Autodesk Inventor part; units mm, degrees
ref_plane "YZ Plane" through (0, 0, 0) normal (1, 0, 0) x (0, 1, 0)
ref_plane "XZ Plane" through (0, 0, 0) normal (0, 1, 0) x (-1, 0, 0)
ref_plane "XY Plane" through (0, 0, 0) normal (0, 0, 1) x (1, 0, 0)
sketch "Sketch1" plane through (0, 0, 0) normal (0, 1, 0) x (-1, 0, 0)
  arc A0 (10, 0) -> (-10, 0) centre (0, 0) ccw
  circle A1 centre (0, 0) radius 5
  line L0 (-10, 0) -> (-10, -100)
  line L1 (-10, -100) -> (10, -100)
  line L2 (10, -100) -> (10, 0)
  dimension "d1" = 10
  dimension "d2" = 100
  dimension "d12" = 20
extrude "Extrusion1" add sketch "Sketch1" along normal blind 80
sketch "Sketch2" plane through (10, 0, -100) normal (0, 0, -1) x (-1, 0, 0)
  line L0 (20, 0) -> (20, 80)
  line L1 (0, 20) -> (20, 20)
  line L2 (20, 20) -> (20, 60)
  line L3 (20, 60) -> (0, 60)
  line L4 (0, 60) -> (0, 20)
  line L5 (0, 20) -> (20, 60) construction
  line L6 (20, 20) -> (0, 60) construction
  point P0 (10, 0)
  point P1 (10, 40)
  dimension "d5" = 40
extrude "Extrusion2" add sketch "Sketch2" along normal blind 40
sketch "Sketch3" plane through (-10, 60, -100) normal (0, 1, 0) x (1, 0, 0)
  circle A0 centre (10, 26.3827) radius 5
  point P0 (10, -100)
  dimension "d8" = 10
extrude "Extrusion3" cut sketch "Sketch3" against normal blind 40
fillet "Fillet1" radius 2 22 edges at (0, 80, 10) (10, 80, -50) (-10, 80, -50) (10, 0, -50) (-10, 0, -50) (0, 0, 10) (-10, 70, -100) (0, 80, -100) (10, 70, -100) (-10, 10, -100) (10, 10, -100) (0, 0, -100) (0, 60, -100) (0, 20, -100) (10, 40, -140) (-10, 40, -140) (0, 20, -140) (10, 20, -120) (-10, 20, -120) (10, 60, -120) (-10, 60, -120) (0, 60, -140)
properties part number "Link1"
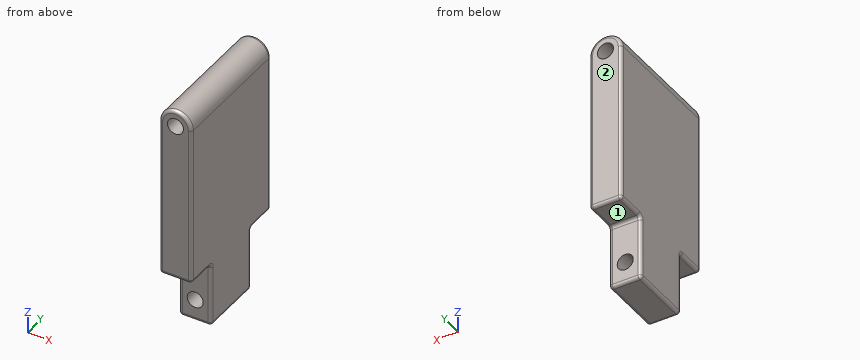
CAD build for the part. Positions are in the model's coordinates, mm. Face numbers are marked on the shaded views. A direction names the side the tool comes from. Coordinates: 2 decimals unless noted, no trailing zeros. Order: outer loops, then holes, each group sorted by start corner. A loop starts at its lowest first (then second) coordinate and runs counter-clockwise, first axis right, second up. Notation, with made-up numbers: (-1.75, -20) - (10.25, -20) arc R5 cw to (10.25, -14) - close; hole circle Ø11 at (-4.5, -18). An arc over 180 degrees is marked (long way). Use a Markdown table: item, result. Add a question column.
(1) Saw through at C-C (y = 44.5). Give the cut face in (x, z), then the cut area to 3 significant figures.
(2) Saw through at D-D (y = 11.5). Give the cut face in (x, z), then the cut area to 3 significant figures.
(3) Which spindle directions (+Z, -Z, +X, -X, +Y, -Y) get a long thin tool onto all of the face, cutting with end or side? Do the marked faces 1 and 2. Say none if no direction does.
(4) Drill centre lines: line 1 along Z through (x, y) = (0, 26); line 2 along Z through (x, y) = (-4, 41); line 3 along Y through (x, z) = (-3, -109). Where is each one in solid material? Low to high. Write a range as [from, to].
(5) Saw through at B-B (z = -128). Give the cut face in (x, y).
(6) Flat gauge pins, fed straight in: pin 1 (5 mm diameter, centred on x = 1, z = -114.5, fed in from +Y); pin 2 (8 mm diameter, centred on x = 2, y = 66.5, fed in from -Z). Where does each tip first touch, or does it go through?
(7) Saw through at A-A (x = 0). Give the cut face in (y, z), then the cut area to 3 significant figures.
Solved:
| question | item | result |
|---|---|---|
| 1 | outline | (-10, -138) arc R2 ccw to (-8, -140) - (8, -140) arc R2 ccw to (10, -138) - (10, 0) arc R10 ccw to (-10, 0) - close; hole circle Ø10 at (0, -126.38); hole circle Ø10 at (0, 0) |
| 1 | area | 2,800 mm² |
| 2 | outline | (-10, -98) arc R2 ccw to (-8, -100) - (8, -100) arc R2 ccw to (10, -98) - (10, 0) arc R10 ccw to (-10, 0) - close; hole circle Ø10 at (0, 0) |
| 2 | area | 2,080 mm² |
| 3 | face 1 | -Z, +X, -X, +Y |
| 3 | face 2 | +Z, -Z, +X, -X, +Y |
| 4 | line 1 | z = [-140, -131.38], [-121.38, -5], [5, 10] |
| 4 | line 2 | z = [-140, -129.38], [-123.38, -3], [3, 9.17] |
| 4 | line 3 | y = [20, 60] |
| 5 | outline | (-10, 22) arc R2 ccw to (-8, 20) - (-4.73, 20) - (-4.73, 60) - (-8, 60) arc R2 ccw to (-10, 58) - close; (4.73, 20) - (8, 20) arc R2 ccw to (10, 22) - (10, 58) arc R2 ccw to (8, 60) - (4.73, 60) - close |
| 6 | pin 1 | stops at y = 60 |
| 6 | pin 2 | stops at z = -100 |
| 7 | outline | (0, -98) arc R2 ccw to (2, -100) - (18, -100) arc R2 cw to (20, -102) - (20, -121.38) - (60, -121.38) - (60, -102) arc R2 cw to (62, -100) - (78, -100) arc R2 ccw to (80, -98) - (80, -5) - (0, -5) - close; (0, 5) - (80, 5) - (80, 8) arc R2 ccw to (78, 10) - (2, 10) arc R2 ccw to (0, 8) - close; (20, -138) arc R2 ccw to (22, -140) - (58, -140) arc R2 ccw to (60, -138) - (60, -131.38) - (20, -131.38) - close |
| 7 | area | 9,200 mm² |
